```python
from build123d import *

# Parameters (mm, degrees)
F0_W     = 127.5
F0_H     = 75
F0_W_2   = 120
F0_H_2   = 70
F1_DEPTH = 25
F2_W     = 120
F2_H     = 7.5
F3_DEPTH = 70
F4_R     = 2.5
F5_DEPTH = 25


with BuildPart() as f1:
    # F0 (on Top) → F1 (new body)
    with BuildSketch(Plane.XY):
        with Locations((-107.463835, -102.613583)):
            Rectangle(F0_W, F0_H)
        with Locations((-106.213835, -102.613583)):
            Rectangle(F0_W_2, F0_H_2, mode=Mode.SUBTRACT)
    extrude(amount=F1_DEPTH)

    # F2 (on face) → F3 (join)
    with BuildSketch(Plane.XZ.offset(67.613583)):
        with Locations((-106.213835, 3.75)):
            Rectangle(F2_W, F2_H)
    extrude(amount=F3_DEPTH)

    # F4 (on face) → F5 (cut)
    with BuildSketch(Plane(origin=(-171.213835, 0, 0), x_dir=(0, -1, 0), z_dir=(-1, 0, 0))):
        with Locations((97.613583, 16.25)):
            Circle(F4_R)
        with Locations((107.613583, 16.25)):
            Circle(F4_R)
    extrude(amount=-F5_DEPTH, mode=Mode.SUBTRACT)


solid = f1.part
```
Source: CAD feature listing. Evaluate the final solid. Frame: model axes, mm. A direction names the side the tool comes from. Coordinates: 2 decimals unless noted, no trailing zeros. Loops run counter-clockwise (first coordinate to the right, second up) from the corner with the lowest first, then second, coordinate; pieces in that order, holes last. Notation, with made-up numbers: M 53.25,-28.75 L 97.25,-28.75 A36 cw 97.25,8.25 Z; hole C 77.25,3 d4. An arc over 180 degrees is marked long. Use a Markdown table: item, result. Add a question column.
Q1. Section query A-A, the plane z = 16.25. Return loops of the section in (x, y), and give its area (3 significant figures).
Q2. Section query C-C, the plane x = -119.5. Return loops of the section in (y, z).
Q3. Material intervals for L1, parallel to X at y = -124.5, z = 19; L2, parallel to Y at x = -140.5, z = 11.5; L3, parallel to X at y = -96, z = 14.5, sorted ascending.
Q4. First-contact query: pin 1 (3 mm diameter, centred on x = -106, y = -91, fed in from -Z); pin 2 (4 mm diameter, centred on y = -107.61, z = 16.25, fed in from -X). Flat tips, straight axial feed; report the tip coordinate or a pass-through.
Q5. Section query B-B, the plane y = -112.5. Return loops of the section in (x, z), and give its area (3 significant figures).
Q6. Access query for faces 4 (the flat face through (-171.214, -103, 12)), 5 (the flat face through (-107, -137.614, 16)), 6 (the cylindrical face through (-169, -100, 17)). Directions: +Z, -Z, +X, -X, +Y, -Y. A direction counts if a zero-diameter tool reaches every point of the face in a straight line with its end or side. Return the directions, or none.
Q7. Draft query along Y for faces 1 (the flat face through (-43.714, -103, 12)), 2 (the flat face through (-166.214, -103, 16)), 3 (the flat face through (-108, -65.114, 12)). Return one class per face: pulls with the +Y half, pulls with the -Y half, needs draft (parallel to the pull), parting line crosses it, or undercut.
Result:
| question | item | result |
|---|---|---|
| 1 | outline | M -171.21,-140.11 L -43.71,-140.11 L -43.71,-65.11 L -171.21,-65.11 L -171.21,-95.11 L -166.21,-95.11 L -166.21,-67.61 L -46.21,-67.61 L -46.21,-137.61 L -166.21,-137.61 L -166.21,-110.11 L -171.21,-110.11 Z; M -171.21,-105.11 L -166.21,-105.11 L -166.21,-100.11 L -171.21,-100.11 Z |
| 1 | area | 1,110 mm2 |
| 2 | outline | M -140.11,0 L -65.11,0 L -65.11,25 L -67.61,25 L -67.61,7.5 L -137.61,7.5 L -137.61,25 L -140.11,25 Z |
| 3 | L1 | x = -171.21 to -166.21, -46.21 to -43.71 |
| 3 | L2 | y = -140.11 to -137.61, -67.61 to -65.11 |
| 3 | L3 | x = -46.21 to -43.71 |
| 4 | pin 1 | stops at z = 0 |
| 4 | pin 2 | stops at x = -46.21 |
| 5 | outline | M -171.21,0 L -43.71,0 L -43.71,25 L -46.21,25 L -46.21,7.5 L -166.21,7.5 L -166.21,25 L -171.21,25 Z |
| 5 | area | 1,090 mm2 |
| 6 | face 4 | +Z, -Z, -X, +Y, -Y |
| 6 | face 5 | +Z |
| 6 | face 6 | -X |
| 7 | face 1 | needs draft |
| 7 | face 2 | undercut |
| 7 | face 3 | pulls with the +Y half |
